Verification items for the finished model (mm, model axes). Give positions to 0.01 mm unless a question says otherwise; leave off trailing zeros. Order: outer loops, then holes, each group sorted by start corner. A loop starts at its lowest first (then second) coordinate and runs counter-clockwise, first axis right, second up. Notation, with made-up numbers: (-33.5, -25) - (20.5, -25) arc R21 cw to (20.5, 1) - close; hole circle Ø1 at (73, 1.5). An arc over 180 degrees is marked (long way). Answer as a JSON object with one key per item and string values. Group by question number.
(1) Section check D-D (y = 8). Record the boundary of the cut face in (x, z) (3 decimals).
(2) Section check A-A (x = 0). Record the boundary of the cut face in (y, z) (3 decimals).
(3) Section check B-B (z = 2.3). Count the separate pieces of the cut face and the enclosed holes in it, then the cut area to 3 significant figures.
(4) Section check C-C (x = 19.05). Record the boundary of the cut face in (y, z) (1 decimal), then the cut area to 3 significant figures.
(5) Thickness scan on line 1 (Y direction, x = -14, z = 0.2); line 2 (Y direction, x = 15, z = 1.5); line 3 (Y direction, x = 18, z = 1.2). Record the ranges inside material, lowest first.
(6) Depth check by flat-ended pin: pin 1 Ø3 at (x, y) = (6.35, 0) entering from -Z; pin 2 Ø2 at (x, y) = (-6.35, 0) entering from -Z; pin 3 Ø1.5 at (y, z) = (-8.5, 3) entering from +X. Enter the tip coordinate at first touch or a pass-through.
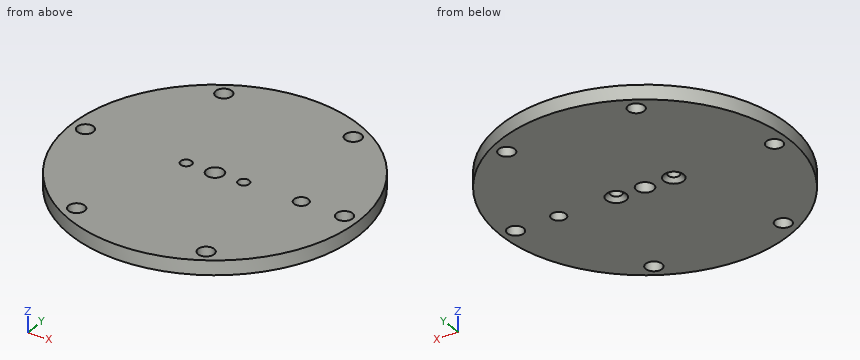
```python
from build123d import *

# Parameters (mm, degrees)
SKETCH1_R                                         = 31.75
BOSS_EXTRUDE1_DEPTH                               = 3.175
CIRPATTERN1_COUNT                                 = 6
SKETCH5_R                                         = 1.905
CUT_EXTRUDE1_DEPTH                                = 4.175
CSK_FOR_2_FLAT_HEAD_MACHINE_SCREW_100_D           = 2.4384
CSK_FOR_2_FLAT_HEAD_MACHINE_SCREW_100_CSINK_D     = 4.3688
CSK_FOR_2_FLAT_HEAD_MACHINE_SCREW_100_CSINK_ANGLE = 100
SKETCH8_R                                         = 1.5875
CUT_EXTRUDE2_DEPTH                                = 4.175


with BuildPart() as part:
    # Sketch1 → Boss-Extrude1 (new body)
    with BuildSketch(Plane.XY):
        Circle(SKETCH1_R)
    extrude(amount=BOSS_EXTRUDE1_DEPTH)

    # Sketch4 → #28 (0.1405) Diameter Hole1 (revolve, cut)
    with BuildSketch(Plane(origin=(14.2875, 24.746675913, 3.175), x_dir=(0, -1, 0), z_dir=(1, 0, 0))):
        Polygon((0, 0), (0, 26.472145646), (1.78435, 25.4), (1.78435, 0), align=None)
    f_28_0_1405_diameter_hole1 = revolve(axis=Axis((14.2875, 24.746675913, 9.525), (0, 0, -1)), mode=Mode.SUBTRACT)

    # CirPattern1: #28 (0.1405) Diameter Hole1 ×6 about axis
    cirpattern1_axis = Axis((0, 0, 0), (0, 0, 1))
    for i in range(1, CIRPATTERN1_COUNT):
        add(f_28_0_1405_diameter_hole1.rotate(cirpattern1_axis, i * 360 / CIRPATTERN1_COUNT), mode=Mode.SUBTRACT)

    # Sketch5 → Cut-Extrude1 (cut, through all)
    with BuildSketch(Plane.XY.offset(3.175)):
        Circle(SKETCH5_R)
    extrude(amount=-CUT_EXTRUDE1_DEPTH, mode=Mode.SUBTRACT)

    # CSK for #2 Flat Head Machine Screw (100)1 (through all)
    with Locations(Plane(origin=(0, 0, 0), x_dir=(-1, 0, 0), z_dir=(0, 0, -1))):
        with Locations((6.35, 0), (-6.35, 0)):
            CounterSinkHole(CSK_FOR_2_FLAT_HEAD_MACHINE_SCREW_100_D / 2, CSK_FOR_2_FLAT_HEAD_MACHINE_SCREW_100_CSINK_D / 2, counter_sink_angle=CSK_FOR_2_FLAT_HEAD_MACHINE_SCREW_100_CSINK_ANGLE)

    # Sketch8 → Cut-Extrude2 (cut, through all)
    with BuildSketch(Plane.XY.offset(3.175)):
        with Locations((19.05, 0)):
            Circle(SKETCH8_R)
    extrude(amount=-CUT_EXTRUDE2_DEPTH, mode=Mode.SUBTRACT)


solid = part.part
```
Solutions:
{
 "1": {"outline": "(-30.726, 0) - (30.726, 0) - (30.726, 3.175) - (-30.726, 3.175) - close"},
 "2": {"outline": "(-31.75, 0) - (-1.905, 0) - (-1.905, 3.175) - (-31.75, 3.175) - close; (1.905, 0) - (31.75, 0) - (31.75, 3.175) - (1.905, 3.175) - close"},
 "3": {"separate pieces": "1", "enclosed holes": "10", "area": "3,080 mm2"},
 "4": {"outline": "(-25.4, 0) - (-1.6, 0) - (-1.6, 3.2) - (-25.4, 3.2) - close; (1.6, 0) - (25.4, 0) - (25.4, 3.2) - (1.6, 3.2) - close", "area": "151 mm2"},
 "5": {"line 1": "y = -28.5 to -26.51, -22.99 to 22.99, 26.51 to 28.5", "line 2": "y = -27.98 to -26.38, -23.11 to 23.11, 26.38 to 27.98", "line 3": "y = -26.15 to -1.19, 1.19 to 26.15"},
 "6": {"pin 1": "stops at z = 0.57", "pin 2": "passes through", "pin 3": "stops at x = 30.79"}
}
